from build123d import *

# Parameters (mm, degrees)
F1_DEPTH = 36.1696
F2_W     = 82.0039
F2_H     = 55.347547
F3_DEPTH = 14.9225


with BuildPart() as f1:
    # F0 (on Top) → F1 (new body)
    with BuildSketch(Plane.XY):
        with BuildLine():
            Line((-15.60195, -68.326), (15.60195, -68.326))
            ThreePointArc((15.60195, -68.326), (33.562462, -60.886512), (41.00195, -42.926))
            Line((41.00195, -42.926), (41.00195, 68.326))
            Line((41.00195, 68.326), (-41.00195, 68.326))
            Line((-41.00195, 68.326), (-41.00195, -42.926))
            ThreePointArc((-41.00195, -42.926), (-33.562462, -60.886512), (-15.60195, -68.326))
        make_face()
    extrude(amount=F1_DEPTH)

    # F2 (on face) → F3 (join)
    with BuildSketch(Plane.XY.offset(36.1696)):
        with Locations((0, 27.673773)):
            Rectangle(F2_W, F2_H)
    extrude(amount=F3_DEPTH)


solid = f1.part
Geometry check sheet. Reference: the model listing, model coordinates, mm. A direction names the side the tool comes from. Coordinates: 2 decimals unless noted, no trailing zeros. Order: outer loops, then holes, each group sorted by start corner. A loop starts at its lowest first (then second) coordinate and runs counter-clockwise, first axis right, second up. Notation, with made-up numbers: (31, 13) - (64, 13) arc R19 cw to (64, 42) - close; hole circle Ø9 at (21, 72.5). An arc over 180 degrees is marked (long way). One line per item, written item: value.
(1) Sectioned sample at B-B (z = 28). Enter the section's corners in (x, y).
Data:
outline: (-41, -42.93) arc R25.4 ccw to (-15.6, -68.33) - (15.6, -68.33) arc R25.4 ccw to (41, -42.93) - (41, 68.33) - (-41, 68.33) - close
(2) Sectioned sample at C-C (y = -25). Enter the section's corners in (x, z), and give its area (3 significant figures).
Data:
outline: (-41, 0) - (41, 0) - (41, 36.17) - (-41, 36.17) - close
area: 2,970 mm^2
(3) Sectioned sample at A-A (x = 9). Enter the section's corners in (y, z), and give its area (3 significant figures).
Data:
outline: (-68.33, 0) - (68.33, 0) - (68.33, 36.17) - (55.35, 36.17) - (55.35, 51.09) - (0, 51.09) - (0, 36.17) - (-68.33, 36.17) - close
area: 5,770 mm^2
(4) Access from +Z, -Z, +X, -X, +Y, -Y to the whole of each face (thin tool, end or side, straight path). Record for faces 1 (the face through (-1, 62, 36.17)), 2 (the face through (-33.759, -60.688, 17.832)), 3 (the face through (-1, 0, 44)).
Data:
face 1: +Z, +X, -X, +Y
face 2: +Z, -Z, -X, -Y
face 3: +Z, +X, -X, -Y
(5) Sectioned sample at D-D (x = 30). Enter the section's corners in (y, z), and give its area (3 significant figures).
Data:
outline: (-63.85, 0) - (68.33, 0) - (68.33, 36.17) - (55.35, 36.17) - (55.35, 51.09) - (0, 51.09) - (0, 36.17) - (-63.85, 36.17) - close
area: 5,610 mm^2
(6) Depth check by flat-ended pin: pin 1 Ø7.5 at (x, z) = (-3.5, 44) entering from -Y; pin 2 Ø4 at (x, y) = (17.5, 60.5) entering from +Z; pin 3 Ø7.5 at (x, z) = (19.5, 43) entering from +Y. Enter the tip coordinate at first touch or a pass-through.
Data:
pin 1: stops at y = 0
pin 2: stops at z = 36.17
pin 3: stops at y = 55.35
(7) Thickness scan on probe 1 along Z at (x, y) = (23, -61.5); probe 2 along Y at (x, z) = (37, 39); probe 3 along Y at (x, z) = (-26, 31.5). Record the ranges inside material, lowest first. Write a range as from..to.
Data:
probe 1: z = 0..36.17
probe 2: y = 0..55.35
probe 3: y = -66.1..68.33
